Verification items for the finished model (mm, model axes). Face numbers are marked on the shaded views. A direction names the side the tool comes from. Round coordinates to 2 decimals unless told otherwise and drop trailing zeros. Write each loop counter-clockwise with the first axis right and the second up, starting at its lowest first coordinate (ties: lowest second). Pieces come first, ordered by that corner, then holes. Notation, with made-up numbers: M 11,79 L 28,79 A31 cw 28,118 Z; hole C 88,-12 d7. An arc over 180 degrees is marked long. Write each question's results on one line, items separated by ' | '.
from build123d import *

# Parameters (mm, degrees)
CROQUIS1_R              = 9.5
CROQUIS1_R_2            = 8.2
SALIENTE_EXTRUIR1_DEPTH = 35
CROQUIS3_R              = 39.137042658
CROQUIS3_R_2            = 38.2
SALIENTE_EXTRUIR2_DEPTH = 130
CROQUIS4_R              = 39.137042658
SALIENTE_EXTRUIR3_DEPTH = 3


with BuildPart() as part:
    # Croquis1 → Saliente-Extruir1 (new body)
    with BuildSketch(Plane(origin=(0, 0, 0), x_dir=(1, 0, 0), z_dir=(0, 1, 0))):
        Circle(CROQUIS1_R)
        Circle(CROQUIS1_R_2, mode=Mode.SUBTRACT)
    extrude(amount=SALIENTE_EXTRUIR1_DEPTH)

    # Croquis2 → Revolución1 (revolve)
    with BuildSketch(Plane.XY):
        Polygon((-9.5, 35), (-39.5, 41), (-39.5, 57), (-38.2, 57), (-38.2, 42.065745074), (-8.2, 36.065745074), (-8.2, 35), align=None)
    revolve(axis=Axis((0, 35, 0), (0, -1, 0)))

    # Croquis3 → Saliente-Extruir2 (add)
    with BuildSketch(Plane(origin=(0, 57, 0), x_dir=(1, 0, 0), z_dir=(0, 1, 0))):
        Circle(CROQUIS3_R)
        Circle(CROQUIS3_R_2, mode=Mode.SUBTRACT)
    extrude(amount=SALIENTE_EXTRUIR2_DEPTH)

    # Croquis4 → Saliente-Extruir3 (add)
    with BuildSketch(Plane(origin=(0, 187, 0), x_dir=(1, 0, 0), z_dir=(0, 1, 0))):
        Circle(CROQUIS4_R)
    extrude(amount=SALIENTE_EXTRUIR3_DEPTH)


solid = part.part
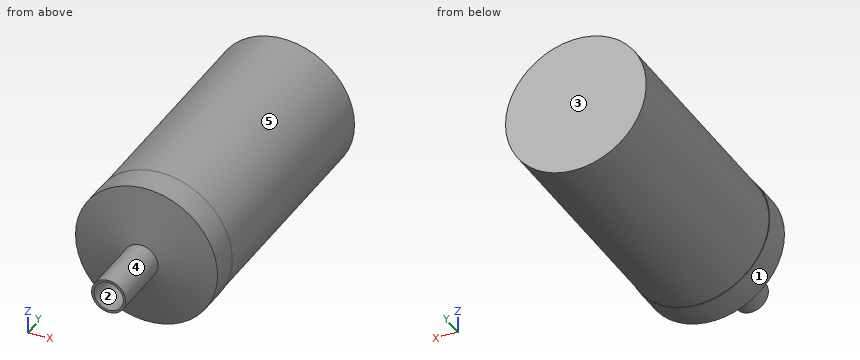
1) Draft check along X on the marked faces 1, 2 and 3. Enter one of: pulls with the +X half, pulls with the -X half, needs draft (parallel to the pull), parting line crosses it, or undercut.
Calculated:
face 1: parting line crosses it | face 2: undercut | face 3: needs draft
2) Sectioned sample at B-B, the plane z = 0. Record the cut outline in (x, y).
Calculated:
outline: M -39.5,41 L -9.5,35 L -9.5,0 L -8.2,0 L -8.2,36.07 L -38.2,42.07 L -38.2,187 L 38.2,187 L 38.2,42.07 L 8.2,36.07 L 8.2,0 L 9.5,0 L 9.5,35 L 39.5,41 L 39.5,57 L 39.14,57 L 39.14,190 L -39.14,190 L -39.14,57 L -39.5,57 Z
3) Sectioned sample at A-A, the plane x = 0. Record the cut outline in (y, z), and give its area (3 significant figures).
Calculated:
outline: M 0,-9.5 L 35,-9.5 L 41,-39.5 L 57,-39.5 L 57,-39.14 L 190,-39.14 L 190,39.14 L 57,39.14 L 57,39.5 L 41,39.5 L 35,9.5 L 0,9.5 L 0,8.2 L 36.07,8.2 L 42.07,38.2 L 187,38.2 L 187,-38.2 L 42.07,-38.2 L 36.07,-8.2 L 0,-8.2 Z | area: 691 mm²
4) Sectioned sample at C-C, the plane y = 77. Record the cut outline in (x, z).
Calculated:
outline: C 0,0 d78.27; hole C 0,0 d76.4
5) Access from +Z, -Z, +X, -X, +Y, -Y to the whole of each face (thin tool, end or side, straight path). Record for the marked faces 4 and 5.
Calculated:
face 4: -Y | face 5: +Y
6) Material ranges on line 1 (Z direction, x = 0, y = 133.5); line 2 (X direction, y = 9, z = 0), recorded low to high. Write a range as [from, to].
Calculated:
line 1: z = [-39.14, -38.2], [38.2, 39.14] | line 2: x = [-9.5, -8.2], [8.2, 9.5]
7) Depth check by flat-ended pin: P1, Ø8, axis at y = 38.5, z = -14.5, coming from the -X side; P2, Ø4, axis at x = -14.5, y = 50, coming from the +Z side; P3, Ø1, axis at x = 2, y = 104, coming from the +Z side. Enter the tip coordinate at first touch or a pass-through.
Calculated:
P1: stops at x = -37.83 | P2: stops at z = 37.47 | P3: stops at z = 39.11
